Verification items for the finished model (mm, model axes). Round coordinates to 2 decimals unless told otherwise and drop trailing zeros. Order: outer loops, then holes, each group sorted by start corner. A loop starts at its lowest first (then second) coordinate and runs counter-clockwise, first axis right, second up. Notation, with made-up numbers: M 80.25,25.25 L 125.25,25.25 A23 cw 125.25,49.25 Z; hole C 24.25,80 d5. An arc over 180 degrees is marked long. Use one line per item in the form item = value. Start each with the question number.
Item 1: Cross-section at A-A on z = 1.2. Enter the section's corners in (x, y).
Item 2: Go/stop test with flat-tipped pins: pin 1 Ø5.5 at (x, y) = (47.5, 22.5) entering from +Z; pin 2 Ø4.5 at (x, y) = (47.5, -22.5) entering from +Z. Record where each tip stops, or that it passes through.
Item 3: Thickness scan on probe 1 along X at (y, z) = (22.5, 0.15); probe 2 along Y at (x, z) = (47.5, 0.3); probe 3 along Y at (x, z) = (-45.5, 1.35). Record the ranges inside material, lowest first. Write a range as [from, to].
Autodesk Inventor part; units mm, degrees
ref_plane "YZ Plane" through (0, 0, 0) normal (1, 0, 0) x (0, 1, 0)
ref_plane "XZ Plane" through (0, 0, 0) normal (0, 1, 0) x (-1, 0, 0)
ref_plane "XY Plane" through (0, 0, 0) normal (0, 0, 1) x (1, 0, 0)
sketch "Sketch1" plane through (0, 0, 0) normal (0, 0, 1) x (1, 0, 0)
  line L0 (-51.5, -26.5) -> (51.5, -26.5)
  line L1 (51.5, -26.5) -> (51.5, 26.5)
  line L2 (51.5, 26.5) -> (-51.5, 26.5)
  line L3 (-51.5, 26.5) -> (-51.5, -26.5)
  line L4 (-51.5, -26.5) -> (51.5, 26.5) construction
  line L5 (51.5, -26.5) -> (-51.5, 26.5) construction
  point P0 (0, 0)
  dimension "d0" = 103
  dimension "d1" = 53
extrude "Extrusion1" add sketch "Sketch1" along normal blind 2
fillet "Fillet1" radius 4 4 edges at (-51.5, -26.5, 1) (-51.5, 26.5, 1) (51.5, -26.5, 1) (51.5, 26.5, 1)
sketch "Sketch2" plane through (0, 0, 2) normal (0, 0, 1) x (1, 0, 0)
  line L0 (-47.5, -22.5) -> (47.5, -22.5) construction
  line L1 (47.5, -22.5) -> (47.5, 22.5) construction
  line L2 (47.5, 22.5) -> (-47.5, 22.5) construction
  line L3 (-47.5, 22.5) -> (-47.5, -22.5) construction
  line L4 (-47.5, -22.5) -> (47.5, 22.5) construction
  line L5 (47.5, -22.5) -> (-47.5, 22.5) construction
  point P0 (0, 0)
  dimension "d5" = 95
  dimension "d6" = 45
hole "Hole1" at (-47.5, 22.5, 2) at (-47.5, -22.5, 2) at (47.5, -22.5, 2) at (47.5, 22.5, 2) direction (0, 0, -1) diameter 3.4 end through all countersink diameter 6.3 countersink angle 90
properties part number "Frontplatte"
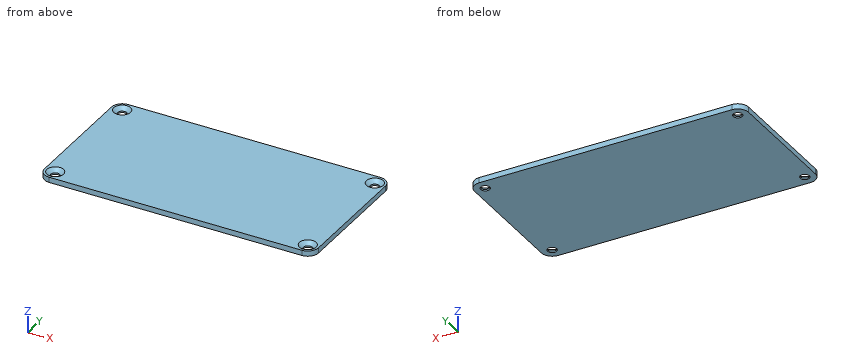
Output values:
q1.outline = M -51.5,-22.5 A4 ccw -47.5,-26.5 L 47.5,-26.5 A4 ccw 51.5,-22.5 L 51.5,22.5 A4 ccw 47.5,26.5 L -47.5,26.5 A4 ccw -51.5,22.5 Z; hole C -47.5,-22.5 d4.7; hole C -47.5,22.5 d4.7; hole C 47.5,-22.5 d4.7; hole C 47.5,22.5 d4.7
q2.pin_1 = 1.6
q2.pin_2 = 1.1
q3.probe_1 = [-51.5, -49.2], [-45.8, 45.8], [49.2, 51.5]
q3.probe_2 = [-26.5, -24.2], [-20.8, 20.8], [24.2, 26.5]
q3.probe_3 = [-26.5, -24], [-21, 21], [24, 26.5]
